Autodesk Inventor part; units mm, degrees
ref_plane "YZ Plane" through (0, 0, 0) normal (1, 0, 0) x (0, 1, 0)
ref_plane "XZ Plane" through (0, 0, 0) normal (0, 1, 0) x (-1, 0, 0)
ref_plane "XY Plane" through (0, 0, 0) normal (0, 0, 1) x (1, 0, 0)
sketch "Sketch1" plane through (0, 0, 0) normal (0, 0, 1) x (1, 0, 0)
  line L0 (-149.86, 0) -> (87.9475, 0)
  line L1 (0, -137.1561) -> (0, 141.8112)
  line L2 (11.7901, -97.3036) -> (11.7901, 101.9587) construction
  circle A0 centre (0, 0) radius 50.8 construction
  circle A1 centre (0, 0) radius 17.4625
  line L3 (1.105, 69.85) -> (-10.1317, 69.85)
  line L4 (10.0665, 66.149) -> (38.0865, 38.2455)
  line L5 (-10.1317, -69.85) -> (1.105, -69.85)
  line L6 (10.0665, -66.149) -> (38.0865, -38.2455)
  arc A2 (38.0865, -38.2455) -> (38.0865, 38.2455) centre (0, 0) ccw
  circle A3 centre (-76.2, 0) radius 14.2875
  arc A4 (-91.6211, 36.5689) -> (-91.6211, -36.5689) centre (-76.2, 0) ccw
  line L7 (-15.0665, 68.8521) -> (-91.6211, 36.5689)
  line L8 (-15.0665, -68.8521) -> (-91.6211, -36.5689)
  line L9 (-63.5889, 6.715) -> (-63.5889, -6.715) construction
  arc A5 (-10.1317, 69.85) -> (-15.0665, 68.8521) centre (-10.1317, 57.15) ccw
  arc A6 (10.0665, 66.149) -> (1.105, 69.85) centre (1.105, 57.15) ccw
  arc A7 (1.105, -69.85) -> (10.0665, -66.149) centre (1.105, -57.15) ccw
  arc A8 (-15.0665, -68.8521) -> (-10.1317, -69.85) centre (-10.1317, -57.15) ccw
  point P0 (11.7901, -97.3036)
  point P1 (11.7901, 101.9587)
  point P2 (46.1798, 0)
  point P3 (6.35, 69.85)
  point P4 (-12.7, 69.85)
  point P5 (6.35, -69.85)
  dimension "d9" = 101.6
  dimension "d10" = 34.925
  dimension "d12" = 69.85
  dimension "d15" = 19.05
  dimension "d16" = 3.175
  dimension "d19" = 28.575
  dimension "d20" = 25.4
  dimension "d22" = 6.35
  dimension "d23" = 6.35
  dimension "d24" = 12.7
  dimension "d25" = 76.2
extrude "Extrusion1" add sketch "Sketch1" along normal mid plane 6.35 contours A4 L7 A5 L3 L1 A1 L0 A3 | L0 A3 A1 L1 L5 A8 L8 A4 | L1 L3 A6 L4 A2 L0 A1 | A1 L0 A2 L6 A7 L5 L1
properties part number "full plate"
Check sheet for the modelled part. Datum: model origin and axes. Units: mm. Give positions to 0.01 mm unless a question says otherwise; leave off trailing zeros. Order: outer loops, then holes, each group sorted by start corner. A loop starts at its lowest first (then second) coordinate and runs counter-clockwise, first axis right, second up. Notation, with made-up numbers: (-27, -2) -> (22, -2) arc R32 ccw to (22, 28) -> close; hole circle Ø7 at (86.5, -9). An arc over 180 degrees is marked (long way). Return JSON: item names as keys, results as strings.
1. Cross-section at D-D, the plane y = 34. Record the cut outline in (x, z) (3 decimals).
From the geometry:
{"outline": "(-96.672, -3.175) -> (41.92, -3.175) -> (41.92, 3.175) -> (-96.672, 3.175) -> close"}
2. Cross-section at B-B, the plane y = 0. Record the cut outline in (x, z) (1 decimal), plus the area to 3 significant figures.
From the geometry:
{"outline": "(-115.9, -3.2) -> (-90.5, -3.2) -> (-90.5, 3.2) -> (-115.9, 3.2) -> close; (-61.9, -3.2) -> (-17.5, -3.2) -> (-17.5, 3.2) -> (-61.9, 3.2) -> close; (17.5, -3.2) -> (54, -3.2) -> (54, 3.2) -> (17.5, 3.2) -> close", "area": "675 mm^2"}
3. Cross-section at C-C, the plane x = -76.2. Record the cut outline in (y, z) (1 decimal).
From the geometry:
{"outline": "(-43.1, -3.2) -> (-14.3, -3.2) -> (-14.3, 3.2) -> (-43.1, 3.2) -> close; (14.3, -3.2) -> (43.1, -3.2) -> (43.1, 3.2) -> (14.3, 3.2) -> close"}
4. Mould release check, pull along X, two halves, no side actions. Record for faces 1 (the cylindrical face through (53.97, 0.6, -0.04)), 2 (the cylindrical face through (-13.858, 10.626, -0.044)), 3 (the flat face through (-52.808, 52.936, -0.044)): +X half, -X half, draft (parallel to the pull), parting line (faces both ways), or undercut.
From the geometry:
{"face 1": "+X half", "face 2": "undercut", "face 3": "-X half"}
5. Material ranges on probe 1 along X at (y, z) = (0, -0.25) (1 decimal); probe 2 along Y at (x, z) = (-1, 2.5); probe 3 along Y at (x, z) = (0, -1.25), recorded low to high. Write a range as [from, to].
From the geometry:
{"probe 1": "[-115.9, -90.5], [-61.9, -17.5], [17.5, 54]", "probe 2": "[-69.85, -17.43], [17.43, 69.85]", "probe 3": "[-69.85, -17.46], [17.46, 69.85]"}
6. Go/stop test with flat-tipped pins: P1, Ø1, axis at y = 54.5, z = 1.5, coming from the +X side; P2, Ø2, axis at x = -27.5, z = 2, coming from the -Y side. Record where each tip stops, or that it passes through.
From the geometry:
{"P1": "x = 22.27", "P2": "y = -64.03"}
7. Cross-section at A-A, the plane z = 0. Count the separate pieces of the cut face and the enclosed holes in it, plus the area to 3 significant figures.
From the geometry:
{"separate pieces": "1", "enclosed holes": "2", "area": "15,000 mm^2"}
